```python
from build123d import *

# Parameters (mm, degrees)
SKETCH2_R          = 1.25
CUT_EXTRUDE1_DEPTH = 19.25
FILLET1_R          = 2
SKETCH3_R          = 2.5
CUT_EXTRUDE2_DEPTH = 13.25
SKETCH4_R          = 5.1
CUT_EXTRUDE3_DEPTH = 6


with BuildPart() as part:
    # Sketch1 → Revolve1 (revolve)
    with BuildSketch(Plane(origin=(0, 0, 0), x_dir=(1, 0, 0), z_dir=(0, 1, 0))):
        Polygon((-6.130434783, 14.45), (6.626387667, 14.45), (10.619565217, 11.440924884), (10.619565217, 4), (14.619565217, 4), (14.619565217, 0), (13.372742768, 0), (-6.130434783, 0), (-7.630434783, 0), (-7.630434783, 18.25), (-6.130434783, 18.25), align=None)
    revolve(axis=Axis((-12.391304348, 0, 0), (1, 0, 0)))

    # Sketch2 → Cut-Extrude1 (cut, through all)
    with BuildSketch(Plane(origin=(10.619565217, 0, 0), x_dir=(0, 0, -1), z_dir=(1, 0, 0))):
        with Locations((0, 9.5)):
            Circle(SKETCH2_R)
        with Locations((6.717514421, 6.717514421)):
            Circle(SKETCH2_R)
        with Locations((9.5, 0)):
            Circle(SKETCH2_R)
        with Locations((6.717514421, -6.717514421)):
            Circle(SKETCH2_R)
        with Locations((0, -9.5)):
            Circle(SKETCH2_R)
        with Locations((-6.717514421, -6.717514421)):
            Circle(SKETCH2_R)
        with Locations((-9.5, 0)):
            Circle(SKETCH2_R)
        with Locations((-6.717514421, 6.717514421)):
            Circle(SKETCH2_R)
    extrude(amount=-CUT_EXTRUDE1_DEPTH, mode=Mode.SUBTRACT)

    # Fillet1
    fillet1_edges = [part.edges().sort_by_distance(p)[0] for p in [
        (14.619565217, 0, 4),
    ]]
    fillet(fillet1_edges, radius=FILLET1_R)

    # Sketch3 → Cut-Extrude2 (cut)
    with BuildSketch(Plane.ZY.offset(7.630434783)):
        with Locations((0, 9.5)):
            Circle(SKETCH3_R)
        with Locations((6.717514421, 6.717514421)):
            Circle(SKETCH3_R)
        with Locations((9.5, 0)):
            Circle(SKETCH3_R)
        with Locations((6.717514421, -6.717514421)):
            Circle(SKETCH3_R)
        with Locations((0, -9.5)):
            Circle(SKETCH3_R)
        with Locations((-6.717514421, -6.717514421)):
            Circle(SKETCH3_R)
        with Locations((-9.5, 0)):
            Circle(SKETCH3_R)
        with Locations((-6.717514421, 6.717514421)):
            Circle(SKETCH3_R)
    extrude(amount=-CUT_EXTRUDE2_DEPTH, mode=Mode.SUBTRACT)

    # Sketch4 → Cut-Extrude3 (cut)
    with BuildSketch(Plane.ZY.offset(7.630434783)):
        Circle(SKETCH4_R)
    extrude(amount=-CUT_EXTRUDE3_DEPTH, mode=Mode.SUBTRACT)


solid = part.part
```
Work out the finished part from the listing and answer in its coordinate system (mm). A direction names the side the tool comes from. Coordinates: 2 decimals unless noted, no trailing zeros. Use CSV: the item, a comma, the result in double quotes. Start each with the question number.
(1) Find section A-A, the plane y = 0. State how many separate pieces and enclosed holes the cut face has, then the cut area to 3 significant figures.
(2) Given pin 1 Ø6 at (y, z) = (9.5, 0) entering from -X; pin 2 Ø8 at (x, z) = (1, -10) entering from -Y; pin 3 Ø6 at (x, y) = (-4.5, 3.5) entering from +Z; pin 4 Ø4.5 at (y, z) = (0, -9.5) entering from +X, each flat-ended and moving along its own axis, determine where each tip first touches the part or whether it passes through.
(3) For faces 1 (the face through (5.62, 11, 1)), 2 (the face through (0.337, 12.184, -7.768)), 3 (the face through (8.15, 0.05, -8.25)), determine the directions among +Z, -Z, +X, -X, +Y, -Y from which every point of the face is accessible in a straight line to the end or side of a thin tool.
(4) Consider line 1 (Z direction, x = -1, y = -8.5); line 2 (Y direction, x = 6.75, z = 0); line 3 (Y direction, x = 7.1, z = 9.5). Determine where each line is inside the solid, lowest interval first.
(5) For a pull along Y with two mould halves and no side action, classify faces 4 (the face through (5.62, -1, 8)), 5 (the face through (-6.87, -17.816, 3.956)), 6 (the face through (-7.63, -4, 4)) as +Y half, -Y half, draft (parallel to the pull), parting line (faces both ways), or undercut.
Recorded:
1,separate pieces,"3"
1,enclosed holes,"0"
1,area,"338 mm^2"
2,pin 1,"stops at x = -7.63"
2,pin 2,"stops at y = -13.15"
2,pin 3,"stops at z = 18.22"
2,pin 4,"stops at x = 10.62"
3,face 1,"-X"
3,face 2,"+X"
3,face 3,"+X, -X"
4,line 1,"z = -11.69 to -8.47, -4.96 to -2.29, 2.29 to 4.96, 8.47 to 11.69"
4,line 2,"y = -14.36 to -10.75, -8.25 to 8.25, 10.75 to 14.36"
4,line 3,"y = -10.41 to -1.25, 1.25 to 10.41"
5,face 4,"undercut"
5,face 5,"parting line"
5,face 6,"draft"
